```python
from build123d import *

# Parameters (mm, degrees)
SKETCH1_W             = 220
SKETCH1_H             = 60
BOSS_EXTRUDE1_DEPTH   = 6.35
FILLET1_R             = 10
F_3_0MM_DOWEL_HOLE1_D = 3
SKETCH6_R             = 12.5
CUT_EXTRUDE1_DEPTH    = 168.825273722
F_6_0MM_DOWEL_HOLE1_D = 6
F_3_0MM_DOWEL_HOLE2_D = 3
F_5_0MM_DOWEL_HOLE1_D = 5


with BuildPart() as part:
    # Sketch1 → Boss-Extrude1 (new body)
    with BuildSketch(Plane(origin=(0, 0, 0), x_dir=(1, 0, 0), z_dir=(0, 1, 0))):
        with Locations((55, 0)):
            Rectangle(SKETCH1_W, SKETCH1_H)
    extrude(amount=BOSS_EXTRUDE1_DEPTH)

    # Fillet1
    fillet1_edges = [part.edges().sort_by_distance(p)[0] for p in [
        (-55, 3.175, -30),
        (165, 3.175, -30),
        (165, 3.175, 30),
        (-55, 3.175, 30),
    ]]
    fillet(fillet1_edges, radius=FILLET1_R)

    # Ø3.0mm Dowel Hole1 (through all)
    with Locations(Plane(origin=(0, 6.35, 0), x_dir=(1, 0, 0), z_dir=(0, 1, 0))):
        with Locations((-15.5, 15.5), (15.5, 15.5), (15.5, -15.5), (-15.5, -15.5)):
            Hole(F_3_0MM_DOWEL_HOLE1_D / 2)

    # Sketch6 → Cut-Extrude1 (cut, through all)
    with BuildSketch(Plane(origin=(0, 6.35, 0), x_dir=(1, 0, 0), z_dir=(0, 1, 0))):
        with Locations(Location((0, 0, 0), (0, 0, 270))):
            Circle(SKETCH6_R)
    extrude(amount=-CUT_EXTRUDE1_DEPTH, mode=Mode.SUBTRACT)

    # Ø6.0mm Dowel Hole1 (through all)
    with Locations(Plane(origin=(0, 6.35, 0), x_dir=(1, 0, 0), z_dir=(0, 1, 0))):
        with Locations((125, 0)):
            Hole(F_6_0MM_DOWEL_HOLE1_D / 2)

    # Ø3.0mm Dowel Hole2 (through all)
    with Locations(Plane(origin=(0, 0, 0), x_dir=(-1, 0, 0), z_dir=(0, -1, 0))):
        with Locations((-139, 9), (-111, 9), (-111, -9), (-139, -9)):
            Hole(F_3_0MM_DOWEL_HOLE2_D / 2)

    # Ø5.0mm Dowel Hole1 (through all)
    with Locations(Plane(origin=(0, 6.35, 0), x_dir=(1, 0, 0), z_dir=(0, 1, 0))):
        with Locations((20, -25), (90, -25), (90, 25), (20, 25), (-40, -25), (-40, 25)):
            Hole(F_5_0MM_DOWEL_HOLE1_D / 2)


solid = part.part
```
Could you check a few things on this model? Use its own coordinates, in mm. Round coordinates to 2 decimals unless told otherwise and drop trailing zeros. Loops run counter-clockwise (first coordinate to the right, second up) from the corner with the lowest first, then second, coordinate; pieces in that order, holes last. Notation, with made-up numbers: (47, 38.5) -> (82, 38.5) arc R25 ccw to (82, 56.5) -> close; hole circle Ø3 at (89, 13). An arc over 180 degrees is marked (long way). One line per question, with ' | ' between items.
(1) If I drill on probe 1 along Z at (x, y) = (-15.5, 3.25); probe 2 along Z at (x, y) = (139, 2.75); probe 3 along Z at (x, y) = (-0.5, 2.5), over which ranges is the centre line in solid material (lowest first)?
Model answer:
probe 1: z = -30 to -17, -14 to 14, 17 to 30 | probe 2: z = -30 to -10.5, -7.5 to 7.5, 10.5 to 30 | probe 3: z = -30 to -12.49, 12.49 to 30
(2) For pin 1 Ø6 at (x, z) = (90, 25) entering from -Y; pin 2 Ø5.5 at (x, z) = (125, 0) entering from +Y, each with a flat end and sliding along its axis, tell me the tip position at first contact or that it passes through.
Model answer:
pin 1: stops at y = 0 | pin 2: passes through
(3) If we section it at B-B on z = -25: List the corners of the cut face in (x, y) for me, and give its area (3 significant figures).
Model answer:
outline: (-53.66, 0) -> (-42.5, 0) -> (-42.5, 6.35) -> (-53.66, 6.35) -> close; (-37.5, 0) -> (17.5, 0) -> (17.5, 6.35) -> (-37.5, 6.35) -> close; (22.5, 0) -> (87.5, 0) -> (87.5, 6.35) -> (22.5, 6.35) -> close; (92.5, 0) -> (163.66, 0) -> (163.66, 6.35) -> (92.5, 6.35) -> close | area: 1,280 mm^2
(4) If we section it at C-C on x = 125: List the corners of the cut face in (y, z) for me, and give its area (3 significant figures).
Model answer:
outline: (0, -30) -> (6.35, -30) -> (6.35, -3) -> (0, -3) -> close; (0, 3) -> (6.35, 3) -> (6.35, 30) -> (0, 30) -> close | area: 343 mm^2
(5) If we section it at A-A on x = 20: List the corners of the cut face in (y, z) for me.
Model answer:
outline: (0, -30) -> (6.35, -30) -> (6.35, -27.5) -> (0, -27.5) -> close; (0, -22.5) -> (6.35, -22.5) -> (6.35, 22.5) -> (0, 22.5) -> close; (0, 27.5) -> (6.35, 27.5) -> (6.35, 30) -> (0, 30) -> close
(6) If we section it at D-D on y = 5: Count the separate pieces of the cut face and the enclosed holes in it, and give its area (3 significant figures).
Model answer:
separate pieces: 1 | enclosed holes: 16 | area: 12,400 mm^2
(7) Thinking about a two-plate mould opening in Z: for faces 1 (the face through (21.84, 3.13, -26.69)), 2 (the face through (-52.15, 3.22, 26.99)), 3 (the face through (54, 3, -30)), which applies, released by +Z, released by -Z, zero draft, split by the parting line, or undercut?
Model answer:
face 1: undercut | face 2: released by +Z | face 3: released by -Z
